from build123d import *

# Parameters (mm, degrees)
SKETCH2_R           = 16
SKETCH2_R_2         = 2
BOSS_EXTRUDE1_DEPTH = 3
SKETCH3_R           = 8
SKETCH3_R_2         = 4
BOSS_EXTRUDE2_DEPTH = 10
SKETCH4_R           = 2
CUT_EXTRUDE1_DEPTH  = 59


with BuildPart() as part:
    # Sketch2 → Boss-Extrude1 (new body)
    with BuildSketch(Plane(origin=(0, 0, 0), x_dir=(1, 0, 0), z_dir=(0, 1, 0))):
        Circle(SKETCH2_R)
        with Locations((0, 12)):
            Circle(SKETCH2_R_2, mode=Mode.SUBTRACT)
        with Locations((-12, 0)):
            Circle(SKETCH2_R_2, mode=Mode.SUBTRACT)
        with Locations((12, 0)):
            Circle(SKETCH2_R_2, mode=Mode.SUBTRACT)
    extrude(amount=BOSS_EXTRUDE1_DEPTH)

    # Sketch3 → Boss-Extrude2 (add)
    with BuildSketch(Plane(origin=(0, 3, 0), x_dir=(1, 0, 0), z_dir=(0, 1, 0))):
        Circle(SKETCH3_R)
        Circle(SKETCH3_R_2, mode=Mode.SUBTRACT)
    extrude(amount=BOSS_EXTRUDE2_DEPTH)

    # Sketch4 → Cut-Extrude1 (cut)
    with BuildSketch(Plane(origin=(0, 3, 0), x_dir=(1, 0, 0), z_dir=(0, 1, 0))):
        with Locations((0, -12)):
            Circle(SKETCH4_R)
    extrude(amount=-CUT_EXTRUDE1_DEPTH, mode=Mode.SUBTRACT)


solid = part.part
Input: part model. Units: mm. Frame: model coordinates. A direction names the side the tool comes from. Give positions to 0.01 mm unless a question says otherwise; leave off trailing zeros. Write each loop counter-clockwise with the first axis right and the second up, starting at its lowest first coordinate (ties: lowest second). Pieces come first, ordered by that corner, then holes.
Q1. Pull-direction query (X, two-part tool) for faces 1 (the face through (-3.47, 1.48, 15.62)), 2 (the face through (10.4, 1.5, 1.2)), 3 (the face through (0, 0, 0)); classes: pulls with the +X half, pulls with the -X half, needs draft (parallel to the pull), parting line crosses it, or undercut.
Q2. Section B-B, the plane y = 2. Output: boundary loops of the cut face in (x, z), plus the area to 3 significant figures.
Q3. Section A-A, the plane x = 0. Output: boundary loops of the cut face in (y, z).
Q4. Section D-D, the plane x = 12. Output: boundary loops of the cut face in (y, z).
Q5. Material intervals for probe 1 along Z at (x, y) = (0, 1.35); probe 2 along X at (y, z) = (8, 0), sorted ascending.
Q6. Set-up query: faces 4 (the face through (-4, 13, 2)), 5 (the face through (-3.8, 3, -7.3)). Return all of +Z, -Z, +X, -X, +Y, -Y with unobstructed straight access to the full face (end or side cutting, diameter ignored); none if empty.
Q7. Section C-C, the plane z = -12. Output: boundary loops of the cut face in (x, y), plus the area to 3 significant figures.
Q8. First-contact query: P1, Ø4, axis at x = 1, z = 0.5, coming from the +Y side; P2, Ø1.5, axis at x = 2.5, y = 2, coming from the -Z side; P3, Ø6, axis at x = 6.5, y = 10, coming from the +Z side. Flat tips, straight axial feed; report the tip coordinate or a pass-through.
Filled in:
1. face 1: parting line crosses it
1. face 2: undercut
1. face 3: needs draft
2. outline: circle Ø32 at (0, 0); hole circle Ø4 at (-12, 0); hole circle Ø4 at (0, -12); hole circle Ø4 at (0, 12); hole circle Ø4 at (12, 0)
2. area: 754 mm2
3. outline: (0, -16) - (3, -16) - (3, -14) - (0, -14) - close; (0, -10) - (3, -10) - (3, -8) - (13, -8) - (13, -4) - (3, -4) - (3, 4) - (13, 4) - (13, 8) - (3, 8) - (3, 10) - (0, 10) - close; (0, 14) - (3, 14) - (3, 16) - (0, 16) - close
4. outline: (0, -10.58) - (3, -10.58) - (3, -2) - (0, -2) - close; (0, 2) - (3, 2) - (3, 10.58) - (0, 10.58) - close
5. probe 1: z = -16 to -14, -10 to 10, 14 to 16
5. probe 2: x = -8 to -4, 4 to 8
6. face 4: +Z, -Z, +X, -X, +Y
6. face 5: +Y
7. outline: (-10.58, 0) - (-2, 0) - (-2, 3) - (-10.58, 3) - close; (2, 0) - (10.58, 0) - (10.58, 3) - (2, 3) - close
7. area: 51.5 mm2
8. P1: stops at y = 3
8. P2: stops at z = -15.9
8. P3: stops at z = 7.19
